```python
from build123d import *

# Parameters (mm, degrees)
SKETCH1_W           = 28.575
SKETCH1_H           = 15.875
SKETCH1_R           = 1.5875
BOSS_EXTRUDE1_DEPTH = 9.525
FILLET1_R           = 1.5875
SKETCH2_W           = 3.175
SKETCH2_H           = 4.7625
BOSS_EXTRUDE2_DEPTH = 2.38125
FILLET2_R           = 0.762
SKETCH3_W           = 0.79375
SKETCH3_H           = 6.35
BOSS_EXTRUDE3_DEPTH = 11.1125
FILLET3_R           = 1.5875
SKETCH4_W           = 3.175
SKETCH4_H           = 0.09921875
CUT_EXTRUDE1_DEPTH  = 0.09921875


with BuildPart() as part:
    # Sketch1 → Boss-Extrude1 (new body)
    with BuildSketch(Plane.XY):
        Rectangle(SKETCH1_W, SKETCH1_H)
        with Locations(Location((11.90625, 5.55625, 0), (0, 0, 180))):
            Circle(SKETCH1_R, mode=Mode.SUBTRACT)
        with Locations(Location((-11.90625, -5.55625, 0), (0, 0, 180))):
            Circle(SKETCH1_R, mode=Mode.SUBTRACT)
    extrude(amount=BOSS_EXTRUDE1_DEPTH)

    # Fillet1
    fillet1_edges = [part.edges().sort_by_distance(p)[0] for p in [
        (-14.2875, 7.9375, 4.7625),
        (14.2875, 7.9375, 4.7625),
        (14.2875, -7.9375, 4.7625),
        (-14.2875, -7.9375, 4.7625),
    ]]
    fillet(fillet1_edges, radius=FILLET1_R)

    # Sketch2 → Boss-Extrude2 (add)
    with BuildSketch(Plane(origin=(0, 7.9375, 0), x_dir=(1, 0, 0), z_dir=(0, 1, 0))):
        with Locations((-9.525, -4.7625)):
            Rectangle(SKETCH2_W, SKETCH2_H)
    extrude(amount=BOSS_EXTRUDE2_DEPTH)

    # Fillet2
    fillet2_edges = [part.edges().sort_by_distance(p)[0] for p in [
        (-11.1125, 10.31875, 4.7625),
        (-7.9375, 10.31875, 4.7625),
    ]]
    fillet(fillet2_edges, radius=FILLET2_R)

    # Sketch3 → Boss-Extrude3 (add)
    with BuildSketch(Plane(origin=(0, -7.9375, 0), x_dir=(-1, 0, 0), z_dir=(0, -1, 0))):
        with Locations((-1.5875, -4.7625)):
            Rectangle(SKETCH3_W, SKETCH3_H)
    extrude(amount=BOSS_EXTRUDE3_DEPTH)

    # Fillet3
    fillet3_edges = [part.edges().sort_by_distance(p)[0] for p in [
        (1.5875, -19.05, 1.5875),
        (1.5875, -19.05, 7.9375),
    ]]
    fillet(fillet3_edges, radius=FILLET3_R)

    # Sketch4 → Cut-Extrude1 (cut)
    with BuildSketch(Plane.XY.offset(7.14375)):
        with Locations((-9.525, 8.681640625)):
            Rectangle(SKETCH4_W, SKETCH4_H)
    cut_extrude1 = extrude(amount=-CUT_EXTRUDE1_DEPTH, mode=Mode.SUBTRACT)

    # Mirror1: Cut-Extrude1 across plane
    add(cut_extrude1.mirror(Plane.XY.offset(4.7625)), mode=Mode.SUBTRACT)


solid = part.part
```
Verification items for the finished model (mm, model axes). A direction names the side the tool comes from. Round coordinates to 2 decimals unless told otherwise and drop trailing zeros. Order: outer loops, then holes, each group sorted by start corner. A loop starts at its lowest first (then second) coordinate and runs counter-clockwise, first axis right, second up. Notation, with made-up numbers: (58.5, 40) -> (106.5, 40) arc R35 cw to (106.5, 72) -> close; hole circle Ø7 at (46, 60). An arc over 180 degrees is marked (long way). Put each result on its own line as item: value. Start each with the question number.
(1) Depth check by flat-ended pin: pin 1 Ø6 at (x, y) = (4, -13) entering from -Z; pin 2 Ø0.5 at (x, y) = (-9.5, 9.5) entering from +Z; pin 3 Ø12 at (x, y) = (6, -14.5) entering from +Z. Enter the tip coordinate at first touch or a pass-through.
(2) Material ranges on line 1 along X through (y, z) = (5.5, 8.5); line 2 along X through (y, z) = (-5.5, 5.5); line 3 along Y through (x, z) = (8, 7.25), recorded low to high.
(3) Section check B-B (x = 12). Enter the section's corners in (y, z) (1 decimal).
(4) Section check D-D (y = -16.25). Enter the section's corners in (x, z), then the cut area to 3 significant figures.
(5) Draft check along X on faces 1 (the face through (13.492, 5.486, 4.696)), 2 (the face through (-10, 10.319, 5)), 3 (the face through (1.984, -13, 5)). Enter one of: +X half, -X half, draft (parallel to the pull), parting line (faces both ways), or undercut.
(6) Section check C-C (z = 9). State how many separate pieces and enclosed holes the cut face has, then the cut area to 3 significant figures.
(7) Section check A-A (y = 4.5). Enter the section's corners in (x, z) (1 decimal).
(8) Tool access check on faces 4 (the face through (-7.938, 9, 5)), 5 (the face through (-11.112, 9, 5)), 6 (the face through (-10, 10, 7.144)). Record the directions out of +Z, -Z, +X, -X, +Y, -Y that give a thin tool (end or side, any length) a straight path to the whole face; none if there is none.
Completed:
1. pin 1: stops at z = 1.59
1. pin 2: stops at z = 7.14
1. pin 3: stops at z = 7.94
2. line 1: x = -14.29 to 10.32, 13.49 to 14.29
2. line 2: x = -14.29 to -13.49, -10.32 to 14.29
2. line 3: y = -7.94 to 7.94
3. outline: (-7.9, 0) -> (4, 0) -> (4, 9.5) -> (-7.9, 9.5) -> close; (7.1, 0) -> (7.9, 0) -> (7.9, 9.5) -> (7.1, 9.5) -> close
4. outline: (1.19, 1.59) -> (1.98, 1.59) -> (1.98, 7.94) -> (1.19, 7.94) -> close
4. area: 5.04 mm2
5. face 1: undercut
5. face 2: draft
5. face 3: +X half
6. separate pieces: 1
6. enclosed holes: 2
6. area: 436 mm2
7. outline: (-14.3, 0) -> (10.7, 0) -> (10.7, 9.5) -> (-14.3, 9.5) -> close; (13.1, 0) -> (14.3, 0) -> (14.3, 9.5) -> (13.1, 9.5) -> close
8. face 4: +Z, -Z, +X, +Y
8. face 5: +Z, -Z, -X, +Y
8. face 6: +Z, +X, -X, +Y
